Build history of the part. All positions in model axes, mm. Give positions to 0.01 mm unless a question says otherwise; leave off trailing zeros. Write each loop counter-clockwise with the first axis right and the second up, starting at its lowest first coordinate (ties: lowest second). Pieces come first, ordered by that corner, then holes. Notation, with made-up numbers: (70, 30) -> (85, 30) arc R17 ccw to (85, 36) -> close; hole circle Ø4 at (21, -27). An arc over 180 degrees is marked (long way). Write item = value, one per line. Start each with the question number.
Q1. Saw through at B-B, the plane y = 1.1. Give the number of separate pieces and of enclosed holes in the cut face, then the cut area to 3 significant figures.
Q2. Wall check: line 1 (Z direction, x = 42.5, y = 1.15); line 2 (X direction, y = 2.55, z = -180); line 3 (Z direction, x = 69.5, y = 1.35). Give the ranges that are in metal, low to high.
Q3. Saw through at A-A, the plane z = -182.5. List the corners of the cut face in (x, y) (3 decimals), then the cut area to 3 significant figures.
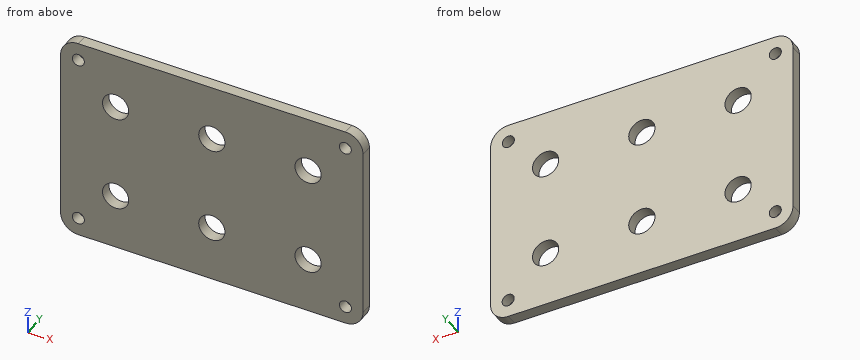
from build123d import *

# Parameters (mm, degrees)
SKETCH1_R           = 3.700636789
SKETCH1_R_2         = 3.700638134
SKETCH1_R_3         = 3.700635443
SKETCH1_R_4         = 1.700388108
SKETCH1_R_5         = 1.700390127
SKETCH1_R_6         = 1.700391472
BOSS_EXTRUDE1_DEPTH = 3.175


with BuildPart() as part:
    # Sketch1 → Boss-Extrude1 (new body)
    with BuildSketch(Plane(origin=(0, 0, 0), x_dir=(1, 0, 0), z_dir=(0, 1, 0))):
        with BuildLine():
            Line((107.487861946, 137.336384548), (32.134526478, 137.336384548))
            add(Edge.make_bspline(
                [(32.134526478, 137.336384548), (29.396970169, 137.336384548), (27.177997625, 139.555359784), (27.177997625, 142.292908018)],
                knots=[1, 1, 1, 1, 2, 2, 2, 2], degree=3))
            Line((27.177997625, 142.292908018), (27.177997625, 190.3800568))
            add(Edge.make_bspline(
                [(27.177997625, 190.3800568), (27.177997625, 193.117610417), (29.396970169, 195.336585653), (32.134526478, 195.336585653)],
                knots=[3, 3, 3, 3, 4, 4, 4, 4], degree=3))
            Line((32.134526478, 195.336585653), (107.487861946, 195.336585653))
            add(Edge.make_bspline(
                [(107.487861946, 195.336585653), (110.225420945, 195.336585653), (112.444385416, 193.1176158), (112.444385416, 190.3800568)],
                knots=[5, 5, 5, 5, 6, 6, 6, 6], degree=3))
            Line((112.444385416, 190.3800568), (112.444385416, 142.292918784))
            add(Edge.make_bspline(
                [(112.444385416, 142.292918784), (112.444385416, 139.555359784), (110.225420945, 137.336384548), (107.487861946, 137.336384548)],
                knots=[7, 7, 7, 7, 8, 8, 8, 8], degree=3))
        make_face()
        with Locations(Location((42.679056729, 179.835523857, 0), (0, 0, 270))):
            Circle(SKETCH1_R, mode=Mode.SUBTRACT)
        with Locations(Location((69.811194212, 179.835523857, 0), (0, 0, 270))):
            Circle(SKETCH1_R_2, mode=Mode.SUBTRACT)
        with Locations(Location((96.946860226, 179.835523857, 0), (0, 0, 270))):
            Circle(SKETCH1_R_3, mode=Mode.SUBTRACT)
        with Locations(Location((42.679056729, 152.837440961, 0), (0, 0, 270))):
            Circle(SKETCH1_R, mode=Mode.SUBTRACT)
        with Locations(Location((69.811194212, 152.837440961, 0), (0, 0, 270))):
            Circle(SKETCH1_R_2, mode=Mode.SUBTRACT)
        with Locations(Location((96.946860226, 152.837440961, 0), (0, 0, 270))):
            Circle(SKETCH1_R_3, mode=Mode.SUBTRACT)
        with Locations(Location((32.180389311, 190.337721152, 0), (0, 0, 270))):
            Circle(SKETCH1_R_4, mode=Mode.SUBTRACT)
        with Locations(Location((32.180389311, 142.338781618, 0), (0, 0, 270))):
            Circle(SKETCH1_R_5, mode=Mode.SUBTRACT)
        with Locations(Location((107.445530335, 142.285856339, 0), (0, 0, 270))):
            Circle(SKETCH1_R_6, mode=Mode.SUBTRACT)
        with Locations(Location((107.494913625, 190.38710848, 0), (0, 0, 270))):
            Circle(SKETCH1_R_6, mode=Mode.SUBTRACT)
    extrude(amount=BOSS_EXTRUDE1_DEPTH)


solid = part.part
Report:
q1.separate_pieces = 1
q1.enclosed_holes = 10
q1.area = 4,630 mm2
q2.line_1 = -195.34 to -183.53, -176.14 to -156.53, -149.14 to -137.34
q2.line_2 = 27.18 to 38.98, 46.38 to 66.11, 73.51 to 93.25, 100.64 to 112.44
q2.line_3 = -195.34 to -183.52, -176.15 to -156.52, -149.15 to -137.34
q3.outline = (27.178, 0) -> (40.111, 0) -> (40.111, 3.175) -> (27.178, 3.175) -> close; (45.247, 0) -> (67.243, 0) -> (67.243, 3.175) -> (45.247, 3.175) -> close; (72.379, 0) -> (94.379, 0) -> (94.379, 3.175) -> (72.379, 3.175) -> close; (99.515, 0) -> (112.444, 0) -> (112.444, 3.175) -> (99.515, 3.175) -> close
q3.area = 222 mm2
